```python
from build123d import *

# Parameters (mm, degrees)
IZIM1_R                     = 30
IZIM1_R_2                   = 25
IZIM1_R_3                   = 40
Y_KSEKLIK_EKSTR_ZYON1_DEPTH = 50


with BuildPart() as part:
    # Çizim1 → Yükseklik-Ekstrüzyon1 (new body)
    with BuildSketch(Plane.XY):
        with BuildLine():
            Line((200, 20), (200, 60))
            ThreePointArc((200, 60), (211.715728753, 88.284271247), (240, 100))
            Line((240, 100), (710, 100))
            ThreePointArc((710, 100), (738.284271247, 88.284271247), (750, 60))
            Line((750, 60), (750, 20))
            ThreePointArc((750, 20), (755.857864376, 5.857864376), (770, 0))
            Line((770, 0), (930, 0))
            ThreePointArc((930, 0), (944.142135624, 5.857864376), (950, 20))
            Line((950, 20), (950, 180))
            ThreePointArc((950, 180), (944.142135624, 194.142135624), (930, 200))
            Line((930, 200), (750, 200))
            ThreePointArc((750, 200), (551.290675458, 246.959096298), (405.571126809, 389.984847569))
            ThreePointArc((405.571126809, 389.984847569), (398.249452654, 397.316133393), (388.241879306, 400))
            Line((388.241879306, 400), (220, 400))
            ThreePointArc((220, 400), (205.857864376, 405.857864376), (200, 420))
            Line((200, 420), (200, 480))
            ThreePointArc((200, 480), (194.142135624, 494.142135624), (180, 500))
            Line((180, 500), (20, 500))
            ThreePointArc((20, 500), (5.857864376, 494.142135624), (0, 480))
            Line((0, 480), (0, 20))
            ThreePointArc((0, 20), (5.857864376, 5.857864376), (20, 0))
            Line((20, 0), (180, 0))
            ThreePointArc((180, 0), (194.142135624, 5.857864376), (200, 20))
        make_face()
        with Locations((100, 400)):
            Circle(IZIM1_R, mode=Mode.SUBTRACT)
        with Locations((100, 100)):
            Circle(IZIM1_R, mode=Mode.SUBTRACT)
        with Locations((350, 250)):
            Circle(IZIM1_R_2, mode=Mode.SUBTRACT)
        with Locations((850, 100)):
            Circle(IZIM1_R_3, mode=Mode.SUBTRACT)
    extrude(amount=Y_KSEKLIK_EKSTR_ZYON1_DEPTH)


solid = part.part
```
Input: part model. Units: mm. Frame: model coordinates. A direction names the side the tool comes from. Give positions to 0.01 mm unless a question says otherwise; leave off trailing zeros. Order: outer loops, then holes, each group sorted by start corner. A loop starts at its lowest first (then second) coordinate and runs counter-clockwise, first axis right, second up. Notation, with made-up numbers: M 59,-6.75 L 79,-6.75 A24 cw 79,14.25 Z; hole C 58,75.5 d1. An arc over 180 degrees is marked long. One line per question, with ' | ' between items.
1) Section C-C on x = 100. Output: boundary loops of the cut face in (y, z).
Filled in:
outline: M 0,0 L 70,0 L 70,50 L 0,50 Z; M 130,0 L 370,0 L 370,50 L 130,50 Z; M 430,0 L 500,0 L 500,50 L 430,50 Z
2) Section D-D on x = 350. Output: boundary loops of the cut face in (y, z), and give its area (3 significant figures).
Filled in:
outline: M 100,0 L 225,0 L 225,50 L 100,50 Z; M 275,0 L 400,0 L 400,50 L 275,50 Z | area: 12,500 mm2
3) Contact query for flat-ended pins moving along their axis: P1, Ø15, axis at x = 852.5, z = 15, coming from the +Y side; P2, Ø10, axis at x = 295.5, z = 13.5, coming from the -Y side; P3, Ø1.5, axis at y = 309, z = 7.5, coming from the +X side; P4, Ø6, axis at x = 475, y = 236.5, coming from the -Z side. Output: stop coordinate, or through.
Filled in:
P1: stops at y = 200 | P2: stops at y = 100 | P3: stops at x = 468.9 | P4: stops at z = 0
4) Ray query, L1, parallel to Y at x = 350, z = 13; L2, parallel to Y at x = 850, z = 32.5; L3, parallel to Y at x = 788.5, z = 34.5. Return the intervals inside material, ascending.
Filled in:
L1: y = 100 to 225, 275 to 400 | L2: y = 0 to 60, 140 to 200 | L3: y = 0 to 200
5) Section B-B on z = 33.5. Output: boundary loops of the cut face in (x, y), and give its area (3 significant figures).
Filled in:
outline: M 0,20 A20 ccw 20,0 L 180,0 A20 ccw 200,20 L 200,60 A40 cw 240,100 L 710,100 A40 cw 750,60 L 750,20 A20 ccw 770,0 L 930,0 A20 ccw 950,20 L 950,180 A20 ccw 930,200 L 750,200 A380 cw 405.57,389.98 A20 ccw 388.24,400 L 220,400 A20 cw 200,420 L 200,480 A20 ccw 180,500 L 20,500 A20 ccw 0,480 Z; hole C 100,100 d60; hole C 100,400 d60; hole C 350,250 d50; hole C 850,100 d80 | area: 242,000 mm2
6) Section A-A on x = 850. Output: boundary loops of the cut face in (y, z).
Filled in:
outline: M 0,0 L 60,0 L 60,50 L 0,50 Z; M 140,0 L 200,0 L 200,50 L 140,50 Z
7) Access query for faces 1 (the face through (841, 200, 25)), 2 (the face through (943.986, 5.703, 24.65)), 3 (the face through (750, 40, 25)). Directions: +Z, -Z, +X, -X, +Y, -Y. A direction counts if a zero-diameter tool reaches every point of the face in a straight line with its end or side. Return the directions, or none.
Filled in:
face 1: +Z, -Z, +X, +Y | face 2: +Z, -Z, +X, -Y | face 3: +Z, -Z, -Y
